from build123d import *

# Parameters (mm, degrees)
EXTRUDE_DEPTH                     = 6
EXTRUDE_ONTO_SKETCH001_ROLL_ANGLE = 90
POCKET_DEPTH                      = 4


with BuildPart() as part:
    # Sketch001 as drawn → Extrude (new)
    with BuildSketch(Plane.XY):
        Polygon((-12.993358, 11.821226), (-12.993358, -12.178774), (11.006642, -12.178774), (11.006642, -6.678774), (-7.493358, -6.678774), (-7.493358, 11.821226), align=None)
    extrude(amount=EXTRUDE_DEPTH)


with BuildPart() as part_1:
    # Extrude onto Sketch001 roll: moved
    add(part.part.rotate(Axis((0, 0, 0), (1, 0, 0)), EXTRUDE_ONTO_SKETCH001_ROLL_ANGLE))


with BuildPart() as part_2:
    # Extrude onto Sketch001 placement: moved
    add(part_1.part)

    # Sketch002 → Pocket (cut)
    with BuildSketch(Plane.XZ.offset(6)):
        Polygon((-10.993358, 9.821226), (-10.993358, -10.178774), (9.006642, -10.178774), (9.006642, -8.678774), (-9.493358, -8.678774), (-9.493358, 9.821226), align=None)
    extrude(amount=-POCKET_DEPTH, mode=Mode.SUBTRACT)


solid = part_2.part
The listing builds one solid part. Answer for the finished solid, in the listing's coordinates (mm). A direction names the side the tool comes from. Round coordinates to 2 decimals unless told otherwise and drop trailing zeros. Loops run counter-clockwise (first coordinate to the right, second up) from the corner with the lowest first, then second, coordinate; pieces in that order, holes last. Notation, with made-up numbers: M 52.5,-5 L 92.5,-5 A12 cw 92.5,12 Z; hole C -31.5,-31 d2. An arc over 180 degrees is marked long. Write each question's results on one line, items separated by ' | '. Start each with the question number.
1) Determine the mould class of faces 4 (the flat face through (-6, -6, -8)), 5 (the flat face through (-10, -4, 9.821)), 6 (the flat face through (2, -3, -6.679)), 7 (the flat face through (-10.993, -4, 0)) for opening direction Z: pulls with the +Z half, pulls with the -Z half, needs draft (parallel to the pull), parting line crosses it, or undercut.
2) Find section A-A on y = -4. Write down the section's boundary in (x, z), plus the area to 3 significant figures.
3) Find section D-D on y = -0.75. Write down the section's boundary in (x, z), plus the area to 3 significant figures.
4) Find section C-C on x = -10.5. Write down the section's boundary in (y, z), plus the area to 3 significant figures.
5) Which of the six approach directions +Z, -Z, +X, -X, +Y, -Y give full straight-line access (tool end or side, diameter ignored) to faces 1 (the flat face through (9.007, -4, -9)), 2 (the flat face through (-7.493, -3, 2)), 3 (the flat face through (-6, 0, -8))?
6) Each of these flat-tipped pins is pushed along its axis until it touches: pin 1 (1.2 mm diameter, centred on x = 4, y = -3.5, fed in from +Z); pin 2 (3 mm diameter, centred on y = -3.5, z = -1.5, fed in from +X). Where does it stop, or does it pass through?
7) Find section B-B on z = -8. Write down the section's boundary in (x, y).
8) Straight lines are drawn through the part: probe 1 along X at (y, z) = (-3, -4.25); probe 2 along Z at (x, y) = (-6.75, -4.5); probe 3 along Y at (x, z) = (-0.25, -10). For each, find the intervals that lie inside material, in ascending order.
Final values:
1) face 4: needs draft | face 5: undercut | face 6: pulls with the +Z half | face 7: undercut
2) outline: M -12.99,-12.18 L 11.01,-12.18 L 11.01,-6.68 L -7.49,-6.68 L -7.49,11.82 L -12.99,11.82 Z; hole M -10.99,-10.18 L 9.01,-10.18 L 9.01,-8.68 L -9.49,-8.68 L -9.49,9.82 L -10.99,9.82 Z | area: 176 mm²
3) outline: M -12.99,-12.18 L 11.01,-12.18 L 11.01,-6.68 L -7.49,-6.68 L -7.49,11.82 L -12.99,11.82 Z | area: 234 mm²
4) outline: M -6,-12.18 L 0,-12.18 L 0,11.82 L -6,11.82 L -6,9.82 L -2,9.82 L -2,-10.18 L -6,-10.18 Z | area: 64.0 mm²
5) face 1: -Y | face 2: +Z, +X, +Y, -Y | face 3: +Z, -Z, +X, -X, +Y
6) pin 1: z = -6.68 | pin 2: x = -7.49
7) outline: M -12.99,-6 L -10.99,-6 L -10.99,-2 L -9.49,-2 L -9.49,-6 L 11.01,-6 L 11.01,0 L -12.99,0 Z
8) probe 1: -12.99 to -10.99, -9.49 to -7.49 | probe 2: -12.18 to -10.18, -8.68 to -6.68 | probe 3: -2 to 0
